Part model, mm, in its own coordinate system. Round coordinates to 2 decimals unless told otherwise and drop trailing zeros. Write each loop counter-clockwise with the first axis right and the second up, starting at its lowest first coordinate (ties: lowest second). Pieces come first, ordered by that corner, then holes.
1) Saw through at A-A on x = 2.75. Write the cut outline in (y, z), and give its area (3 significant figures).
2) Pull direction X, two halves, no side cores. Call faces 1 (the cylindrical face through (1.827, -1.726, 50.558)), 2 (the flat face through (3.437, -2.08, 48.67)), 3 (the flat face through (2, -2.236, 50)): +X half, -X half, draft (parallel to the pull), parting line (faces both ways), or undercut.
3) Saw through at B-B on y = 4.25. Count the separate pieces of the cut face and the enclosed holes in it, and give its area (3 significant figures).
4) Flat gauge pins, fed straight in: pin 1 (4 mm diameter, centred on x = 6.5, z = 49, fed in from -Y); pin 2 (6 mm diameter, centred on x = 20.5, z = 46.5, fed in from -Y); pin 3 (4 mm diameter, centred on y = 4.5, z = 48.5, fed in from +X); pin 4 (5 mm diameter, centred on x = 18, y = 10.5, fed in from -Z). Where does each tip first touch, or does it go through?
5) Drill centre line: L1, parallel to X at y = 0.75, z = 57. Where is it in solid material? Low to high.
```python
from build123d import *

# Parameters (mm, degrees)
EXTRUDE2_DEPTH = 3.175


with BuildPart() as part:
    # Sketch2 → Revolve-Thin2 (revolve)
    with BuildSketch(Plane(origin=(54.9, 0, 50.401640227), x_dir=(-1, 0, 0), z_dir=(0, 0, -1))):
        Polygon((46.764200866, -1.710829687), (46.764200866, 0.8348085), (48.796200866, 0.699341833), (48.796200866, -1.846296354), (54.638200866, -2.23576302), (54.638200866, 2.59023698), (31.778200866, 2.59023698), (31.778200866, -0.71176302), (36.350200866, -1.01656302), (36.350200866, 1.529075166), (38.382200866, 1.3936085), (38.382200866, -1.152029687), (41.557200866, -1.363696354), (41.557200866, 1.181941833), (43.589200866, 1.046475166), (43.589200866, -1.49916302), align=None)
        Polygon((46.763997666, -1.710612489), (46.763997666, 0.835025698), (48.796404066, 0.699531938), (48.796404066, -1.846106249), (54.637997666, -2.235545823), (54.637997666, 2.59003378), (31.778404066, 2.59003378), (31.778404066, -0.711572916), (36.349997666, -1.016345823), (36.349997666, 1.529292364), (38.382404066, 1.393798604), (38.382404066, -1.151839583), (41.556997666, -1.363479156), (41.556997666, 1.182159031), (43.589404066, 1.046665271), (43.589404066, -1.498972916), align=None, mode=Mode.SUBTRACT)
    revolve(axis=Axis((0.261799134, 5.38423698, 50.401640227), (1, 0, 0)))

    # Sketch4 → Extrude2 (add)
    with BuildSketch(Plane.ZY.offset(-0.261595934)):
        with BuildLine():
            Line((42.781423057, 5.38423698), (42.781423057, -2.23598019))
            Line((42.781423057, -2.23598019), (58.021857397, -2.23598019))
            Line((58.021857397, -2.23598019), (58.021857397, 5.38423698))
            Line((58.021857397, 5.38423698), (57.513640227, 5.38423698))
            ThreePointArc((57.513640227, 5.38423698), (50.401640227, -1.72776302), (43.289640227, 5.38423698))
            Line((43.289640227, 5.38423698), (42.781423057, 5.38423698))
        make_face()
    extrude(amount=-EXTRUDE2_DEPTH)


solid = part.part
```
Completed:
1. outline: (-2.24, 42.78) - (5.38, 42.78) - (5.38, 42.95) arc R7.45 ccw to (5.38, 57.86) - (5.38, 58.02) - (-2.24, 58.02) - close; circle Ø5.59 at (5.38, 50.4); hole circle Ø5.59 at (5.38, 50.4); hole (5.38, 42.95) arc R7.45 ccw to (5.38, 57.86) - (5.38, 57.51) arc R7.11 ccw to (5.38, 43.29) - close
1. area: 36.7 mm2
2. face 1: undercut
2. face 2: +X half
2. face 3: draft
3. separate pieces: 2
3. enclosed holes: 2
3. area: 3.83 mm2
4. pin 1: stops at y = -1.93
4. pin 2: stops at y = -0.86
4. pin 3: stops at x = 23.12
4. pin 4: stops at z = 44.59
5. L1: x = 0.26 to 3.44
